```python
from build123d import *

# Parameters (mm, degrees)
SKETCH1_W           = 42
SKETCH1_H           = 20
SKETCH1_R           = 1.95
BOSS_EXTRUDE1_DEPTH = 5
SKETCH2_R           = 1.25
CUT_EXTRUDE1_DEPTH  = 10
CUT_EXTRUDE2_DEPTH  = 10
FILLET1_R           = 1
CHAMFER1_SIZE       = 2


with BuildPart() as part:
    # Sketch1 → Boss-Extrude1 (new body)
    with BuildSketch(Plane.XY):
        with Locations((21, -10)):
            Rectangle(SKETCH1_W, SKETCH1_H)
        with Locations((38.5, -16)):
            Circle(SKETCH1_R, mode=Mode.SUBTRACT)
        with Locations((3.5, -16)):
            Circle(SKETCH1_R, mode=Mode.SUBTRACT)
    extrude(amount=BOSS_EXTRUDE1_DEPTH)

    # Sketch2 → Cut-Extrude1 (cut)
    with BuildSketch(Plane(origin=(0, 0, 0), x_dir=(1, 0, 0), z_dir=(0, 1, 0))):
        with Locations((36, -2.5)):
            Circle(SKETCH2_R)
        with Locations((6, -2.5)):
            Circle(SKETCH2_R)
    extrude(amount=-CUT_EXTRUDE1_DEPTH, mode=Mode.SUBTRACT)

    # Sketch3 → Cut-Extrude2 (cut)
    with BuildSketch(Plane.XY.offset(5)):
        with BuildLine():
            Line((29, -13.990346174), (13, -13.990346174))
            ThreePointArc((13, -13.990346174), (11.585786438, -13.404559737), (11, -11.990346174))
            Line((11, -11.990346174), (11, -5.990346174))
            ThreePointArc((11, -5.990346174), (11.585786438, -4.576132612), (13, -3.990346174))
            Line((13, -3.990346174), (29, -3.990346174))
            ThreePointArc((29, -3.990346174), (30.414213562, -4.576132612), (31, -5.990346174))
            Line((31, -5.990346174), (31, -11.990346174))
            ThreePointArc((31, -11.990346174), (30.414213562, -13.404559737), (29, -13.990346174))
        make_face()
    extrude(amount=-CUT_EXTRUDE2_DEPTH, mode=Mode.SUBTRACT)

    # Fillet1
    fillet1_edges = [part.edges().sort_by_distance(p)[0] for p in [
        (42, -10, 5),
        (21, 0, 5),
        (0, -10, 5),
        (21, -20, 5),
    ]]
    fillet(fillet1_edges, radius=FILLET1_R)

    # Chamfer1
    chamfer1_edges = [part.edges().sort_by_distance(p)[0] for p in [
        (21, -13.990346174, 0),
        (30.414213562, -13.404559737, 0),
        (31, -8.990346174, 0),
        (30.414213562, -4.576132612, 0),
        (21, -3.990346174, 0),
        (11.585786438, -4.576132612, 0),
        (11, -8.990346174, 0),
        (11.585786438, -13.404559737, 0),
        (11.585786438, -13.404559737, 5),
        (21, -13.990346174, 5),
        (30.414213562, -13.404559737, 5),
        (31, -8.990346174, 5),
        (30.414213562, -4.576132612, 5),
        (21, -3.990346174, 5),
        (11.585786438, -4.576132612, 5),
        (11, -8.990346174, 5),
    ]]
    chamfer(chamfer1_edges, length=CHAMFER1_SIZE)


solid = part.part
```
Geometry check sheet. Reference: the model listing, model coordinates, mm. A direction names the side the tool comes from. Round coordinates to 2 decimals unless told otherwise and drop trailing zeros. Order: outer loops, then holes, each group sorted by start corner. A loop starts at its lowest first (then second) coordinate and runs counter-clockwise, first axis right, second up. Notation, with made-up numbers: M 35,-18.5 L 79,-18.5 A14 cw 79,6.5 Z; hole C 39,-26.75 d4. An arc over 180 degrees is marked long. Write item = value, one per line.
Q1. Scan lines: line 1 (X direction, y = -3.5, z = 2.5); line 2 (Y direction, x = 3.5, z = 2.85); line 3 (X direction, y = -7.5, z = 2.5). Record each from-to range of solid material in increasing order.
Answer block:
line_1 = 0 to 4.75, 7.25 to 34.75, 37.25 to 42
line_2 = -20 to -17.95, -14.05 to 0
line_3 = 0 to 4.75, 7.25 to 11, 31 to 34.75, 37.25 to 42
Q2. Set-up check for faces 1 (the cylindrical face through (0.285, -9.86, 4.699)), 2 (the cylindrical face through (35.01, -4.93, 3.26)), 3 (the flat face through (32, -9, 4)), 4 (the flat face through (20.89, -3, 1.01)), 5 (the flat face through (31, -8.9, 2.5)): record each of +Z, -Z, +X, -X, +Y, -Y from which the full face is reachable in a straight line by a thin tool's end or side.
Answer block:
face_1 = +Z, -X, +Y, -Y
face_2 = +Y
face_3 = +Z
face_4 = -Z
face_5 = +Z, -Z
Q3. Section check D-D (y = -17.5). Enter the section's corners in (x, z).
Answer block:
outline = M 0,0 L 2.25,0 L 2.25,5 L 1,5 A1 ccw 0,4 Z; M 4.75,0 L 37.25,0 L 37.25,5 L 4.75,5 Z; M 39.75,0 L 42,0 L 42,4 A1 ccw 41,5 L 39.75,5 Z
Q4. Release check for a two-part mould opening along Y. For faces 6 (the flat face through (21, -20, 2)), 7 (the flat face through (20.89, -3, 3.99)), 8 (the flat face through (0, -10, 2)), 9 (the conical face through (11.024, -4.058, 3.764)) record: released by +Y, released by -Y, zero draft, split by the parting line, or undercut.
Answer block:
face_6 = released by -Y
face_7 = undercut
face_8 = zero draft
face_9 = undercut
Q5. Section check B-B (x = 38.5). Enter the section's corners in (y, z).
Answer block:
outline = M -20,0 L -17.95,0 L -17.95,5 L -19,5 A1 ccw -20,4 Z; M -14.05,0 L 0,0 L 0,4 A1 ccw -1,5 L -14.05,5 Z
Q6. Section check A-A (y = -7.5). Enter the section's corners in (x, z), plus the area to 3 significant figures.
Answer block:
outline = M 0,0 L 9,0 L 11,2 L 11,3 L 9,5 L 1,5 A1 ccw 0,4 Z; M 31,2 L 33,0 L 42,0 L 42,4 A1 ccw 41,5 L 33,5 L 31,3 Z; hole C 6,2.5 d2.5; hole C 36,2.5 d2.5
area = 91.8 mm^2
Q7. Section check C-C (z = 2.5). Enter the section's corners in (x, y), plus the area to 3 significant figures.
Answer block:
outline = M 0,-20 L 42,-20 L 42,0 L 37.25,0 L 37.25,-10 L 34.75,-10 L 34.75,0 L 7.25,0 L 7.25,-10 L 4.75,-10 L 4.75,0 L 0,0 Z; hole C 3.5,-16 d3.9; hole M 11,-11.99 A2 ccw 13,-13.99 L 29,-13.99 A2 ccw 31,-11.99 L 31,-5.99 A2 ccw 29,-3.99 L 13,-3.99 A2 ccw 11,-5.99 Z; hole C 38.5,-16 d3.9
area = 570 mm^2
Q8. Depth check by flat-ended pin: pin 1 Ø2 at (x, z) = (6, 2.5) entering from +Y. Enter the tip coordinate at first touch or a pass-through.
Answer block:
pin_1 = -10
